from build123d import *

# Parameters (mm, degrees)
BOSS_EXTRUDE1_DEPTH  = 4.7625
M4_CLEARANCE_HOLE1_D = 4.5


with BuildPart() as part:
    # Sketch1 → Boss-Extrude1 (new body)
    with BuildSketch(Plane.XY):
        with BuildLine():
            Line((139.473530069, 101.6), (70.133530069, 101.6))
            Line((70.133530069, 101.6), (70.133530069, 105.0097))
            ThreePointArc((70.133530069, 105.0097), (64.633530069, 110.5097), (59.133530069, 105.0097))
            Line((59.133530069, 105.0097), (59.133530069, 101.6))
            Line((59.133530069, 101.6), (-10.206469931, 101.6))
            ThreePointArc((-10.206469931, 101.6), (-11.288333767, 101.542235923), (-12.357895857, 101.36960052))
            Line((-12.357895857, 101.36960052), (-15.912609523, 104.924314185))
            ThreePointArc((-15.912609523, 104.924314185), (-23.690784116, 104.924314185), (-23.690784116, 97.146139592))
            Line((-23.690784116, 97.146139592), (-20.13607045, 93.591425927))
            ThreePointArc((-20.13607045, 93.591425927), (-20.308705854, 92.521863836), (-20.366469931, 91.44))
            Line((-20.366469931, 91.44), (-20.366469931, 39.225226889))
            Line((-20.366469931, 39.225226889), (-23.776169931, 39.225226889))
            ThreePointArc((-23.776169931, 39.225226889), (-29.276169931, 33.725226889), (-23.776169931, 28.225226889))
            Line((-23.776169931, 28.225226889), (-20.366469931, 28.225226889))
            Line((-20.366469931, 28.225226889), (-20.366469931, -28.225226889))
            Line((-20.366469931, -28.225226889), (-23.776169931, -28.225226889))
            ThreePointArc((-23.776169931, -28.225226889), (-29.276169931, -33.725226889), (-23.776169931, -39.225226889))
            Line((-23.776169931, -39.225226889), (-20.366469931, -39.225226889))
            Line((-20.366469931, -39.225226889), (-20.366469931, -91.44))
            ThreePointArc((-20.366469931, -91.44), (-20.308705854, -92.521863836), (-20.13607045, -93.591425927))
            Line((-20.13607045, -93.591425927), (-23.690784116, -97.146139592))
            ThreePointArc((-23.690784116, -97.146139592), (-23.690784116, -104.924314185), (-15.912609523, -104.924314185))
            Line((-15.912609523, -104.924314185), (-12.357895857, -101.36960052))
            ThreePointArc((-12.357895857, -101.36960052), (-11.288333767, -101.542235923), (-10.206469931, -101.6))
            Line((-10.206469931, -101.6), (59.133530069, -101.6))
            Line((59.133530069, -101.6), (59.133530069, -105.0097))
            ThreePointArc((59.133530069, -105.0097), (64.633530069, -110.5097), (70.133530069, -105.0097))
            Line((70.133530069, -105.0097), (70.133530069, -101.6))
            Line((70.133530069, -101.6), (139.473530069, -101.6))
            ThreePointArc((139.473530069, -101.6), (140.555393905, -101.542235923), (141.624955996, -101.36960052))
            Line((141.624955996, -101.36960052), (145.179669661, -104.924314185))
            ThreePointArc((145.179669661, -104.924314185), (152.957844254, -104.924314185), (152.957844254, -97.146139592))
            Line((152.957844254, -97.146139592), (149.403130589, -93.591425927))
            ThreePointArc((149.403130589, -93.591425927), (149.575765992, -92.521863836), (149.633530069, -91.44))
            Line((149.633530069, -91.44), (149.633530069, -39.225226889))
            Line((149.633530069, -39.225226889), (153.043230069, -39.225226889))
            ThreePointArc((153.043230069, -39.225226889), (158.543230069, -33.725226889), (153.043230069, -28.225226889))
            Line((153.043230069, -28.225226889), (149.633530069, -28.225226889))
            Line((149.633530069, -28.225226889), (149.633530069, 28.225226889))
            Line((149.633530069, 28.225226889), (153.043230069, 28.225226889))
            ThreePointArc((153.043230069, 28.225226889), (158.543230069, 33.725226889), (153.043230069, 39.225226889))
            Line((153.043230069, 39.225226889), (149.633530069, 39.225226889))
            Line((149.633530069, 39.225226889), (149.633530069, 91.44))
            ThreePointArc((149.633530069, 91.44), (149.575765992, 92.521863836), (149.403130589, 93.591425927))
            Line((149.403130589, 93.591425927), (152.957844254, 97.146139592))
            ThreePointArc((152.957844254, 97.146139592), (152.957844254, 104.924314185), (145.179669661, 104.924314185))
            Line((145.179669661, 104.924314185), (141.624955996, 101.36960052))
            ThreePointArc((141.624955996, 101.36960052), (140.555393905, 101.542235923), (139.473530069, 101.6))
        make_face()
    extrude(amount=BOSS_EXTRUDE1_DEPTH)

    # M4 Clearance Hole1 (through all)
    with Locations(Plane.XY.offset(4.7625)):
        with Locations((-19.801696819, -101.035226889), (-23.776169931, -33.725226889), (-23.776169931, 33.725226889), (-19.801696819, 101.035226889), (64.633530069, 105.0097), (149.068756958, 101.035226889), (153.043230069, 33.725226889), (153.043230069, -33.725226889), (149.068756958, -101.035226889), (64.633530069, -105.0097)):
            Hole(M4_CLEARANCE_HOLE1_D / 2)


solid = part.part
Source: CAD feature listing. Evaluate the final solid. Frame: model axes, mm. A direction names the side the tool comes from. Give positions to 0.01 mm unless a question says otherwise; leave off trailing zeros. Write each loop counter-clockwise with the first axis right and the second up, starting at its lowest first coordinate (ties: lowest second). Pieces come first, ordered by that corner, then holes. Notation, with made-up numbers: M -11,-32 L 37,-32 A22 ccw 37,-19 Z; hole C -27,75.5 d8. An arc over 180 degrees is marked long. Return JSON: item names as keys, results as strings. Group by question number.
1) Set-up query: faces 1 (the face through (104, -101.6, 2)), 2 (the face through (25, 101.6, 2)), 3 (the face through (149.634, -66, 2)). Return all of +Z, -Z, +X, -X, +Y, -Y with unobstructed straight access to the full face (end or side cutting, diameter ignored); none if empty.
2) Draft query along X for faces 4 (the face through (-29.275, -33.604, 2.348)), 5 (the face through (158.54, 33.6, 2.35)), 6 (the face through (105, 101.6, 2)). Return one class per face: released by +X, released by -X, zero draft, split by the parting line, or undercut.
3) Ray query, L1, parallel to X at y = 35.5, z = 3.45; L2, parallel to Y at x = 148, z = 2.9; L3, parallel to Y at x = 21, z = 2.15. Return the intervals inside material, ascending.
4) Cut plane B-B, the plane y = -12. Output: boundary loops of the cut face in (x, z).
5) First-contact query: pin 1 Ø3.5 at (x, y) = (-19.8, -101.04) entering from -Z; pin 2 Ø1 at (x, z) = (-21.5, 3.5) entering from +Y; pin 3 Ø2.5 at (y, z) = (54, 3.5) entering from -X; pin 4 Ø1.4 at (x, z) = (92, 3.5) entering from -Y. Flat tips, straight axial feed; report the tip coordinate or a pass-through.
6) Cut plane A-A, the plane x = 96. Output: boundary loops of the cut face in (y, z).
7) Cut plane C-C, the plane z = 3.8. Give the number of separate pieces and of enclosed holes in the cut face, then the cut area to 3 significant figures.
Data:
{
 "1": {"face 1": "+Z, -Z, -Y", "face 2": "+Z, -Z, +Y", "face 3": "+Z, -Z, +X"},
 "2": {"face 4": "released by -X", "face 5": "released by +X", "face 6": "undercut"},
 "3": {"L1": "x = -28.98 to -25.16, -22.39 to 151.66, 154.43 to 158.25", "L2": "y = -106.43 to -103.02, -99.06 to 99.06, 103.02 to 106.43", "L3": "y = -101.6 to 101.6"},
 "4": {"outline": "M -20.37,0 L 149.63,0 L 149.63,4.76 L -20.37,4.76 Z"},
 "5": {"pin 1": "passes through", "pin 2": "stops at y = 106.4", "pin 3": "stops at x = -20.37", "pin 4": "stops at y = -101.6"},
 "6": {"outline": "M -101.6,0 L 101.6,0 L 101.6,4.76 L -101.6,4.76 Z"},
 "7": {"separate pieces": "1", "enclosed holes": "10", "area": "35,200 mm²"}
}
